Geometry: final body of the model. Coordinates: model frame, mm. Face numbers are marked on the shaded views. Give positions to 0.01 mm unless a question says otherwise; leave off trailing zeros. Loops run counter-clockwise (first coordinate to the right, second up) from the corner with the lowest first, then second, coordinate; pieces in that order, holes last. Notation, with made-up numbers: (56.25, 37.25) -> (76.25, 37.25) arc R21 cw to (76.25, 73.25) -> close; hole circle Ø8 at (76, 7.25). An arc over 180 degrees is marked (long way). Answer in a Markdown table with one row per item. Add a question column.
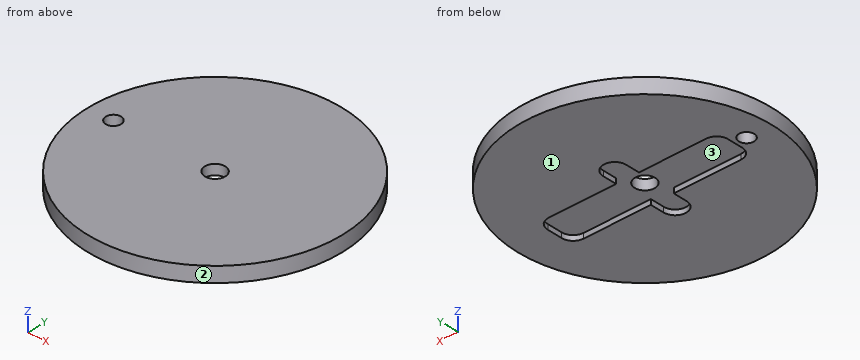
Autodesk Inventor part; units mm, degrees
ref_plane "YZ Plane" through (0, 0, 0) normal (1, 0, 0) x (0, 1, 0)
ref_plane "XZ Plane" through (0, 0, 0) normal (0, 1, 0) x (-1, 0, 0)
ref_plane "XY Plane" through (0, 0, 0) normal (0, 0, 1) x (1, 0, 0)
sketch "Boceto1" plane through (0, 0, 0) normal (0, 0, 1) x (1, 0, 0)
  circle A0 centre (0, 0) radius 25
  dimension "d0" = 50
extrude "Extrusión1" add sketch "Boceto1" along normal blind 3
sketch "Boceto2" plane through (0, 0, 3) normal (0, 0, 1) x (1, 0, 0)
  circle A0 centre (0, 0) radius 2
  dimension "d3" = 4
extrude "Extrusión2" cut sketch "Boceto2" against normal blind 3
sketch "Boceto3" plane through (0, 0, 3) normal (0, 0, 1) x (1, 0, 0)
  circle A0 centre (0, 0) radius 2 construction
  circle A1 centre (0, 0) radius 25 construction
  line L0 (0, 0) -> (-25, 0) construction
  circle A2 centre (0, 0) radius 25 construction
  circle A3 centre (-20, 0) radius 1.5
  dimension "d6" = 3
  dimension "d7" = 20
extrude "Extrusión3" cut sketch "Boceto3" against normal blind 3
sketch "Boceto4" plane through (0, 0, 0) normal (0, 0, -1) x (-1, 0, 0)
  arc A0 (-17.5, -1.5) -> (-15.5, -3.5) centre (-15.5, -1.5) ccw construction
  line L0 (-2, -3.5) -> (-15.5, -3.5) construction
  line L1 (-2, -6.5) -> (-2, -3.5) construction
  arc A1 (-2, -6.5) -> (2, -6.5) centre (0, -6.5) ccw construction
  line L2 (2, -3.5) -> (2, -6.5) construction
  line L3 (15.5, -3.5) -> (2, -3.5) construction
  arc A2 (15.5, -3.5) -> (17.5, -1.5) centre (15.5, -1.5) ccw construction
  line L4 (17.5, 1.5) -> (17.5, -1.5) construction
  arc A3 (17.5, 1.5) -> (15.5, 3.5) centre (15.5, 1.5) ccw construction
  line L5 (2, 3.5) -> (15.5, 3.5) construction
  line L6 (2, 6.5) -> (2, 3.5) construction
  arc A4 (2, 6.5) -> (-2, 6.5) centre (0, 6.5) ccw construction
  line L7 (-2, 3.5) -> (-2, 6.5) construction
  line L8 (-15.5, 3.5) -> (-2, 3.5) construction
  arc A5 (-15.5, 3.5) -> (-17.5, 1.5) centre (-15.5, 1.5) ccw construction
  line L9 (-17.5, -1.5) -> (-17.5, 1.5) construction
  line L10 (0, 8.5) -> (0, -8.5) construction
  line L11 (-17.5, 0) -> (17.5, 0) construction
  line L12 (-2.25, 3.75) -> (-2.25, 6.5)
  arc A6 (2.25, 6.5) -> (-2.25, 6.5) centre (0, 6.5) ccw
  line L13 (2.25, 6.5) -> (2.25, 3.75)
  line L14 (2.25, 3.75) -> (15.5, 3.75)
  arc A7 (17.75, 1.5) -> (15.5, 3.75) centre (15.5, 1.5) ccw
  line L15 (17.75, 1.5) -> (17.75, -1.5)
  arc A8 (15.5, -3.75) -> (17.75, -1.5) centre (15.5, -1.5) ccw
  line L16 (15.5, -3.75) -> (2.25, -3.75)
  line L17 (2.25, -3.75) -> (2.25, -6.5)
  arc A9 (-2.25, -6.5) -> (2.25, -6.5) centre (0, -6.5) ccw
  line L18 (-2.25, -6.5) -> (-2.25, -3.75)
  line L19 (-2.25, -3.75) -> (-15.5, -3.75)
  arc A10 (-17.75, -1.5) -> (-15.5, -3.75) centre (-15.5, -1.5) ccw
  line L20 (-17.75, -1.5) -> (-17.75, 1.5)
  arc A11 (-15.5, 3.75) -> (-17.75, 1.5) centre (-15.5, 1.5) ccw
  line L21 (-15.5, 3.75) -> (-2.25, 3.75)
  point P0 (0, 0)
  point P1 (17.5, -3.5)
  point P2 (0, 0)
  dimension "d10" = 0.25
extrude "Extrusión4" cut sketch "Boceto4" against normal blind 1
properties part number "rueda"
(1) Cut plane B-B on x = 0. Return the cut outline in (y, z), then the cut area to 4 significant figures.
(2) Cut plane D-D on z = 2.3. Return the cut outline in (x, y).
(3) Cut plane C-C on x = -20. Return the cut outline in (y, z).
(4) Draft query along X for the marked faces 1, 2 and 3. Return one class per face: +X half, -X half, draft (parallel to the pull), parting line (faces both ways), or undercut.
(5) Pin query (flat end, axial travel): pin 1 Ø0.5 at (x, z) = (9, 0.5) entering from -Y; pin 2 Ø0.8 at (y, z) = (-5, 0.5) entering from +X; pin 3 Ø1.1 at (x, z) = (12, 0.5) entering from +Y. Return the tip coordinate at first contact, or that it passes through.
(6) Material intervals for line 1 along Y through (x, z) = (0, 1.75); line 2 along X through (y, z) = (-6, 0.4); line 3 along Y through (x, z) = (-16, 0.7), sorted ascending. Write a range as from..to.
(7) Cut plane A-A on y = 0. Return the cut outline in (x, z).
Answer list:
| question | item | result |
|---|---|---|
| 1 | outline | (-25, 0) -> (-8.75, 0) -> (-8.75, 1) -> (-2, 1) -> (-2, 3) -> (-25, 3) -> close; (2, 1) -> (8.75, 1) -> (8.75, 0) -> (25, 0) -> (25, 3) -> (2, 3) -> close |
| 1 | area | 124.5 mm² |
| 2 | outline | circle Ø50 at (0, 0); hole circle Ø3 at (-20, 0); hole circle Ø4 at (0, 0) |
| 3 | outline | (-15, 0) -> (-1.5, 0) -> (-1.5, 3) -> (-15, 3) -> close; (1.5, 0) -> (15, 0) -> (15, 3) -> (1.5, 3) -> close |
| 4 | face 1 | draft |
| 4 | face 2 | parting line |
| 4 | face 3 | undercut |
| 5 | pin 1 | stops at y = -23.42 |
| 5 | pin 2 | stops at x = 24.57 |
| 5 | pin 3 | stops at y = 22.22 |
| 6 | line 1 | y = -25..-2, 2..25 |
| 6 | line 2 | x = -24.27..-2.25, 2.25..24.27 |
| 6 | line 3 | y = -19.21..-3.69, 3.69..19.21 |
| 7 | outline | (-25, 0) -> (-21.5, 0) -> (-21.5, 3) -> (-25, 3) -> close; (-18.5, 0) -> (-17.75, 0) -> (-17.75, 1) -> (-2, 1) -> (-2, 3) -> (-18.5, 3) -> close; (2, 1) -> (17.75, 1) -> (17.75, 0) -> (25, 0) -> (25, 3) -> (2, 3) -> close |
